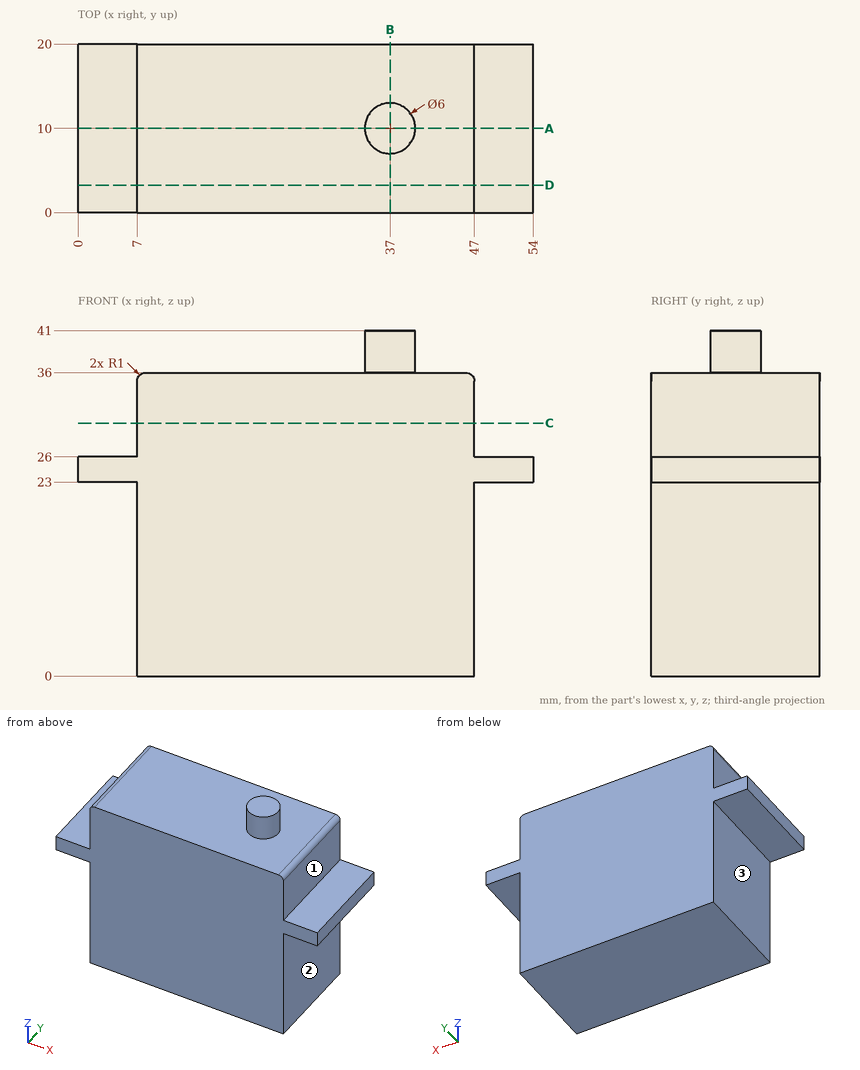
Source: three-view drawing plus pictorial views. Frame: mm from the lowest corner of the part. A direction names the side the tool comes from. Round coordinates to 2 decimals unless told otherwise and drop trailing zeros. Write each loop counter-clockwise with the first axis right and the second up, starting at its lowest first coordinate (ties: lowest second). Pieces come first, ordered by that corner, then holes. Notation, with made-up numbers: M -35,-30.75 L -17,-30.75 A26 cw -17,-4.75 Z; hole C 44.5,-34 d7. An arc over 180 degrees is marked long. One line per item, written item: value. Start each with the question number.
Item 1: Pin query (flat end, axial travel): pin 1 (4 mm diameter, centred on x = 16, z = 9.5, fed in from -Y); pin 2 (7 mm diameter, centred on y = 11.5, z = 31.5, fed in from +X); pin 3 (1.5 mm diameter, centred on x = 6, z = 32, fed in from -Y); pin 4 (6 mm diameter, centred on y = 10, z = 10.5, fed in from -X). Return the tip coordinate at first contact, or that it passes through.
Item 2: Set-up query: the marked faces 1, 2 and 3. Return all of +Z, -Z, +X, -X, +Y, -Y with unobstructed straight access to the full face (end or side cutting, diameter ignored); none if empty.
Item 3: Ray query, L1, parallel to X at y = 11.5, z = 18; L2, parallel to Z at x = 41, y = 8.5; L3, parallel to Z at x = 5, y = 8.75. Return the intervals inside material, ascending. Write a range as from..to.
Item 4: Section query B-B (x = 37). Return the cut outline in (y, z).
Item 5: Section query A-A (y = 10). Return the cut outline in (x, z), plus the area to 3 significant figures.
Item 6: Section query C-C (z = 30). Return the cut outline in (x, y).
Item 7: Section query D-D (y = 3.25). Return the cut outline in (x, z), plus the area to 3 significant figures.
Result set:
1. pin 1: stops at y = 0
1. pin 2: stops at x = 47
1. pin 3: passes through
1. pin 4: stops at x = 7
2. face 1: +Z, +X, +Y, -Y
2. face 2: -Z, +X, +Y, -Y
2. face 3: -Z, -X, +Y, -Y
3. L1: x = 7..47
3. L2: z = 0..36
3. L3: z = 23..26
4. outline: M 0,0 L 20,0 L 20,36 L 13,36 L 13,41 L 7,41 L 7,36 L 0,36 Z
5. outline: M 0,23 L 7,23 L 7,0 L 47,0 L 47,23 L 54,23 L 54,26 L 47,26 L 47,35 A1 ccw 46,36 L 40,36 L 40,41 L 34,41 L 34,36 L 8,36 A1 ccw 7,35 L 7,26 L 0,26 Z
5. area: 1,510 mm²
6. outline: M 7,0 L 47,0 L 47,20 L 7,20 Z
7. outline: M 0,23 L 7,23 L 7,0 L 47,0 L 47,23 L 54,23 L 54,26 L 47,26 L 47,35 A1 ccw 46,36 L 8,36 A1 ccw 7,35 L 7,26 L 0,26 Z
7. area: 1,480 mm²
